```python
from build123d import *

# Parameters (mm, degrees)
EXTRUDE_1_DEPTH     = 7
FILLET_1_R          = 3.5
SKETCH_2_R          = 1.55
CUT_EXTRUDE_1_DEPTH = 16.173990905
FILLET_2_R          = 1.5
FILLET_3_R          = 0.8


# Some blends are built 0.0001 mm under size
with BuildPart() as part:
    # 草图1 → 凸台-拉伸1 (new body)
    with BuildSketch(Plane.XY):
        Polygon((2, -2.5), (2.5, -2.5), (3.5, -2.5), (3.5, 4.5), (-3.5, 4.5), (-3.5, -2.5), (-2.5, -2.5), (1, -2.5), (1, -11.5), (0.5, -11.5), (-1.5, -11.5), (-1.5, -4.5), (-4.5, -4.5), (-5.5, -4.5), (-5.5, 6.5), (5.5, 6.5), (5.5, -4.5), (4.5, -4.5), (4.5, -11.5), (2.5, -11.5), (2, -11.5), align=None)
    extrude(amount=-EXTRUDE_1_DEPTH)

    # 圆角1
    fillet_1_edges = [part.edges().sort_by_distance(p)[0] for p in [
        (3.25, -11.5, 0),
        (3.25, -11.5, -7),
        (-0.25, -11.5, -7),
        (-0.25, -11.5, 0),
    ]]
    fillet(fillet_1_edges, radius=FILLET_1_R - 0.0001)  # a hair under: the kernel refuses the full size

    # 草图2 → 切除-拉伸1 (cut, through all)
    with BuildSketch(Plane.ZY.offset(1.5)):
        with Locations((-3.5, -8)):
            Circle(SKETCH_2_R)
    extrude(amount=-CUT_EXTRUDE_1_DEPTH, mode=Mode.SUBTRACT)

    # 圆角2
    # the kernel refuses this fillet: 1.5 mm, written as the material it adds along each edge
    with BuildSketch(Plane(origin=(4.5, -4.5, 0), x_dir=(1, 0, 0), z_dir=(0, 0, -1))) as fillet_2_piece_1:
        with BuildLine():
            CenterArc((1.5, 1.414213562), FILLET_2_R, 180, 70.528779366)
            Line((0, 1.414213562), (-0.03, 1.414213562))
            Line((-0.03, 1.414213562), (-0.03, 0))
            Line((-0.03, 0), (0, -0.03))
            ThreePointArc((0, -0.03), (0.5, -0.03), (0.99, -0.028284271))
            Line((0.99, -0.028284271), (1, 0))
        make_face()
    extrude(amount=7)

    # 圆角3
    fillet_3_edges = [part.edges().sort_by_distance(p)[0] for p in [
        (-1.5, -6.25005, 0),
        (-3.5, -4.5, 0),
        (-5.5, 1, 0),
        (5.5, 1, 0),
        (5.5, 1, -7),
        (-5.5, 1, -7),
        (-3.5, -4.5, -7),
        (-5.5, 6.5, -3.5),
        (5.5, 6.5, -3.5),
        (-1.5, -6.25005, -7),
        (4.5, -6.957156781, 0),
        (4.5, -6.957156781, -7),
        (4.5, -10.474903023, -5.974903023),
        (4.5, -10.474903023, -1.025096977),
        (-1.5, -10.474903023, -1.025096977),
        (-1.5, -10.474903023, -5.974903023),
        (4.775255129, -5.048188159, 0),
        (4.775255129, -5.048188159, -7),
    ]]
    fillet(fillet_3_edges, radius=FILLET_3_R)


solid = part.part
```
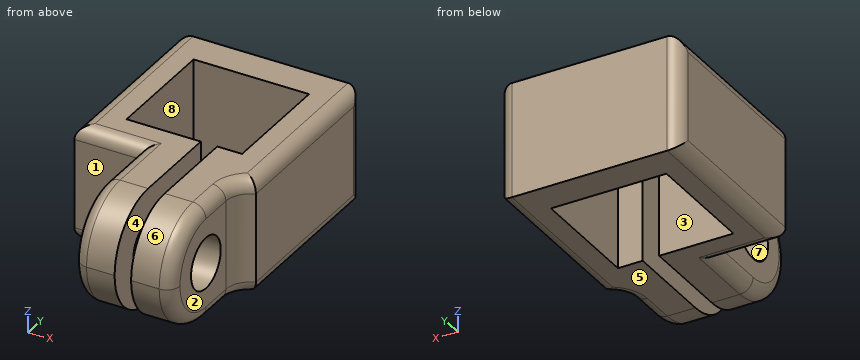
Could you check a few things on this model? Use its own coordinates, in mm. Face numbers are marked on the shaded views. A direction names the side the tool comes from. Round coordinates to 2 decimals unless told otherwise and drop trailing zeros. Loops run counter-clockwise (first coordinate to the right, second up) from the corner with the lowest first, then second, coordinate; pieces in that order, holes last. Notation, with made-up numbers: M 23.5,11.25 L 77.5,11.25 A14 ccw 77.5,21.25 Z; hole C 84,14 d8. An arc over 180 degrees is marked long. Put each result on its own line as item: value.
Q1. Thinking about a two-plate mould opening in Z: for the marked faces 5, 6, 7 and 8, which applies, released by +Z, released by -Z, zero draft, split by the parting line, or undercut?
Check result:
face 5: released by -Z
face 6: released by +Z
face 7: undercut
face 8: zero draft
Q2. Imagine slicing it at D-D (x = -1.75). Write out the boundary of the cut face in (y, z), then the cut area to 3 significant figures.
Check result:
outline: M -4.5,-6.2 A0.8 ccw -3.7,-7 L -2.5,-7 L -2.5,0 L -3.7,0 A0.8 ccw -4.5,-0.8 Z; M 4.5,-7 L 6.5,-7 L 6.5,0 L 4.5,0 Z
area: 27.7 mm2
Q3. Imagine slicing it at C-C (y = -6.75). Write out the boundary of the cut face in (x, z), then the cut area to 3 significant figures.
Check result:
outline: M -1.5,-6.2 A0.8 ccw -0.7,-7 L 1,-7 L 1,-4.42 L -1.5,-4.42 Z; M -1.5,-2.58 L 1,-2.58 L 1,0 L -0.7,0 A0.8 ccw -1.5,-0.8 Z; M 2,-7 L 3.7,-7 A0.8 ccw 4.5,-6.2 L 4.5,-4.42 L 2,-4.42 Z; M 2,-2.58 L 4.5,-2.58 L 4.5,-0.8 A0.8 ccw 3.7,0 L 2,0 Z
area: 25.3 mm2
Q4. Imagine slicing it at B-B (x = 0). State how many separate pieces and enclosed holes the cut face has, then the cut area to 3 significant figures.
Check result:
separate pieces: 2
enclosed holes: 1
area: 64.2 mm2
Q5. On a 3-axis mill with a long thin cutter (end or side, diameter ignored), from which of +Z, -Z, +X, -X, +Y, -Y can I reach the whole of each face in a straight line? I mean the marked faces 1, 2, 3 and 4. Say none if no direction works.
Check result:
face 1: +Z, -Z, -X, -Y
face 2: +Z, -Z, +X, -Y
face 3: +Z, -Z
face 4: +Z, -Z, -Y
Q6. Imagine slicing it at A-A (y = -1.5). Write out the boundary of the cut face in (x, z).
Check result:
outline: M -5.5,-6.2 A0.8 ccw -4.7,-7 L -3.5,-7 L -3.5,0 L -4.7,0 A0.8 ccw -5.5,-0.8 Z; M 3.5,-7 L 4.7,-7 A0.8 ccw 5.5,-6.2 L 5.5,-0.8 A0.8 ccw 4.7,0 L 3.5,0 Z
Q7. I need wall thicknesses on probe 1 along Y at (x, z) = (0.35, -3.5); probe 2 along X at (y, z) = (3.25, -3.75); probe 3 along X at (y, z) = (-6.25, -1.5). Which ranges of each line are inside material? Lowest first, please.
Check result:
probe 1: -11.5 to -9.55, -6.45 to -2.5, 4.5 to 6.5
probe 2: -5.5 to -3.5, 3.5 to 5.5
probe 3: -1.5 to 1, 2 to 4.5
Q8. For pin 1 (3 mm diameter, centred on y = -9, z = -2.5, fed in from +X); pin 2 (2 mm diameter, centred on y = -8.5, z = -4, fed in from -X); pin 3 (1.2 mm diameter, centred on x = -4.5, z = -2.5, fed in from -Y); pin 4 (2.5 mm diameter, centred on y = -8, z = -3.5, fed in from -X), each with a flat end and sliding along its axis, tell me the tip position at first contact or that it passes through.
Check result:
pin 1: x = 4.5
pin 2: x = -1.5
pin 3: y = -4.5
pin 4: through
